Geometry check sheet. Reference: the model listing, model coordinates, mm. Face numbers are marked on the shaded views. A direction names the side the tool comes from. Round coordinates to 2 decimals unless told otherwise and drop trailing zeros. Order: outer loops, then holes, each group sorted by start corner. A loop starts at its lowest first (then second) coordinate and runs counter-clockwise, first axis right, second up. Notation, with made-up numbers: (71, -24) -> (76, -24) arc R37 cw to (76, 13) -> close; hole circle Ø1 at (-30.75, -15). An arc over 180 degrees is marked (long way). Use a Markdown table: item, result. Add a question column.
Item 1: Sectioned sample at C-C, the plane y = 12. Record the cut outline in (x, z), and give its area (3 significant figures).
Item 2: Gauge pin test, flat ends, axial feed: pin 1 Ø20.5 at (x, z) = (-65, 112.58) entering from -Y; pin 2 Ø3 at (y, z) = (97.5, 22.5) entering from -X; pin 3 Ø8 at (x, y) = (53, 109) entering from -Z. Record the tip position at first contact, or that the pin passes through.
Item 3: Sectioned sample at D-D, the plane y = 115. Record the cut outline in (x, z), and give its area (3 significant figures).
Item 4: Sectioned sample at A-A, the plane z = 0. State how many separate pieces and enclosed holes the cut face has, and give its area (3 significant figures).
Item 5: Set-up check for the marked faces 1 and 2: record each of +Z, -Z, +X, -X, +Y, -Y from which the full face is reachable in a straight line by a thin tool's end or side.
Item 6: Material ranges on probe 1 along X at (y, z) = (13.25, 0); probe 2 along Y at (x, z) = (24.5, 107); probe 3 along X at (y, z) = (37, 2) (3 decimals), recorded low to high. Write a range as [from, to].
Item 7: Sectioned sample at B-B, the plane x = 0. Record the cut outline in (y, z).
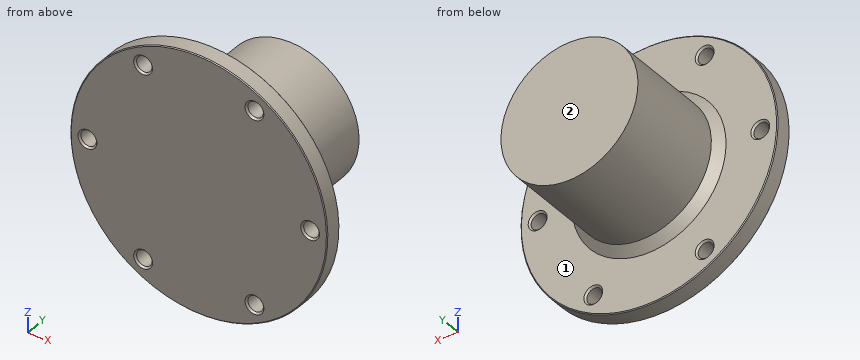
from build123d import *

# Parameters (mm, degrees)
SKIZZE1_R                       = 150
SKIZZE1_R_2                     = 9
AUFSATZ_LINEAR_AUSTRAGEN1_DEPTH = 20
SKIZZE3_R                       = 80
AUFSATZ_LINEAR_AUSTRAGEN2_DEPTH = 130
FASE1_SIZE                      = 1
FASE2_SIZE                      = 10
FASE3_SIZE                      = 2


with BuildPart() as part:
    # Skizze1 → Aufsatz-Linear austragen1 (new body)
    with BuildSketch(Plane(origin=(0, 0, 0), x_dir=(1, 0, 0), z_dir=(0, 1, 0))):
        with Locations(Location((0, 0, 0), (0, 0, 270))):
            Circle(SKIZZE1_R)
        with Locations(Location((130, 0, 0), (0, 0, 270))):
            Circle(SKIZZE1_R_2, mode=Mode.SUBTRACT)
        with Locations(Location((65, -112.583302492, 0), (0, 0, 270))):
            Circle(SKIZZE1_R_2, mode=Mode.SUBTRACT)
        with Locations(Location((-65, -112.583302492, 0), (0, 0, 270))):
            Circle(SKIZZE1_R_2, mode=Mode.SUBTRACT)
        with Locations(Location((-130, 0, 0), (0, 0, 270))):
            Circle(SKIZZE1_R_2, mode=Mode.SUBTRACT)
        with Locations(Location((-65, 112.583302492, 0), (0, 0, 270))):
            Circle(SKIZZE1_R_2, mode=Mode.SUBTRACT)
        with Locations(Location((65, 112.583302492, 0), (0, 0, 270))):
            Circle(SKIZZE1_R_2, mode=Mode.SUBTRACT)
    extrude(amount=AUFSATZ_LINEAR_AUSTRAGEN1_DEPTH)

    # Skizze3 → Aufsatz-Linear austragen2 (add)
    with BuildSketch(Plane(origin=(0, 20, 0), x_dir=(1, 0, 0), z_dir=(0, 1, 0))):
        with Locations(Location((0, 0, 0), (0, 0, 270))):
            Circle(SKIZZE3_R)
    extrude(amount=AUFSATZ_LINEAR_AUSTRAGEN2_DEPTH)

    # Fase1
    fase1_edges = [part.edges().sort_by_distance(p)[0] for p in [
        (0, 0, -150),
        (0, 20, -150),
    ]]
    chamfer(fase1_edges, length=FASE1_SIZE)

    # Fase2
    fase2_edges = [part.edges().sort_by_distance(p)[0] for p in [
        (0, 20, -80),
    ]]
    chamfer(fase2_edges, length=FASE2_SIZE)

    # Fase3
    fase3_edges = [part.edges().sort_by_distance(p)[0] for p in [
        (-65, 0, 103.583302492),
        (-65, 20, 103.583302492),
        (-130, 0, -9),
        (-130, 20, -9),
        (-65, 0, -121.583302492),
        (-65, 20, -121.583302492),
        (65, 0, -121.583302492),
        (65, 20, -121.583302492),
        (130, 0, -9),
        (130, 20, -9),
        (65, 0, 103.583302492),
        (65, 20, 103.583302492),
    ]]
    chamfer(fase3_edges, length=FASE3_SIZE)


solid = part.part
Found:
| question | item | result |
|---|---|---|
| 1 | outline | circle Ø300 at (0, 0); hole circle Ø18 at (-130, 0); hole circle Ø18 at (-65, -112.58); hole circle Ø18 at (-65, 112.58); hole circle Ø18 at (65, -112.58); hole circle Ø18 at (65, 112.58); hole circle Ø18 at (130, 0) |
| 1 | area | 69,200 mm2 |
| 2 | pin 1 | stops at y = 0.75 |
| 2 | pin 2 | stops at x = -77.19 |
| 2 | pin 3 | stops at z = -63.24 |
| 3 | outline | circle Ø160 at (0, 0) |
| 3 | area | 20,100 mm2 |
| 4 | separate pieces | 3 |
| 4 | enclosed holes | 0 |
| 4 | area | 26,200 mm2 |
| 5 | face 1 | +Y |
| 5 | face 2 | +Z, -Z, +X, -X, +Y |
| 6 | probe 1 | x = [-150, -139], [-121, 121], [139, 150] |
| 6 | probe 2 | y = [0, 20] |
| 6 | probe 3 | x = [-79.975, 79.975] |
| 7 | outline | (0, -149) -> (1, -150) -> (19, -150) -> (20, -149) -> (20, -90) -> (30, -80) -> (150, -80) -> (150, 80) -> (30, 80) -> (20, 90) -> (20, 149) -> (19, 150) -> (1, 150) -> (0, 149) -> close |
